Verification items for the finished model (mm, model axes). A direction names the side the tool comes from. Coordinates: 2 decimals unless noted, no trailing zeros. Write each loop counter-clockwise with the first axis right and the second up, starting at its lowest first coordinate (ties: lowest second). Pieces come first, ordered by that corner, then holes. Notation, with made-up numbers: (-20.75, 55) -> (33.25, 55) arc R14 cw to (33.25, 59) -> close; hole circle Ø11 at (78.5, 77). An arc over 180 degrees is marked (long way). Answer in a Markdown table with one row per item.
```python
from build123d import *

# Parameters (mm, degrees)
SKETCH_1_R      = 13.5
EXTRUDE_1_DEPTH = 2.5


with BuildPart() as part:
    # 草图1 → 凸台-拉伸1 (new body)
    with BuildSketch(Plane(origin=(0, 0, 0), x_dir=(1, 0, 0), z_dir=(0, 1, 0))):
        with Locations(Location((0, 0, 0), (0, 0, 90))):
            Circle(SKETCH_1_R)
        Polygon((0, -6.119912853), (5.3, -3.059956427), (5.3, 3.059956427), (0, 6.119912853), (-5.3, 3.059956427), (-5.3, -3.059956427), align=None, mode=Mode.SUBTRACT)
    extrude(amount=EXTRUDE_1_DEPTH)


solid = part.part
```
1. Sectioned sample at A-A, the plane z = 0. Record the cut outline in (x, y).
Findings below:
| item | result |
|---|---|
| outline | (-13.5, 0) -> (-5.3, 0) -> (-5.3, 2.5) -> (-13.5, 2.5) -> close; (5.3, 0) -> (13.5, 0) -> (13.5, 2.5) -> (5.3, 2.5) -> close |
2. Sectioned sample at C-C, the plane x = -1.5. Record the cut outline in (y, z).
Findings below:
| item | result |
|---|---|
| outline | (0, -13.42) -> (2.5, -13.42) -> (2.5, -5.25) -> (0, -5.25) -> close; (0, 5.25) -> (2.5, 5.25) -> (2.5, 13.42) -> (0, 13.42) -> close |
3. Release check for a two-part mould opening along Z. For faces 3 (the face through (-2.687, 1.232, 4.569)), 4 (the face through (6, 2.5, 0)), 5 (the face through (13.18, 1.23, 2.93)), 6 (the face through (-5.3, 1, 0)) record: released by +Z, released by -Z, zero draft, split by the parting line, or undercut.
Findings below:
| item | result |
|---|---|
| face 3 | undercut |
| face 4 | zero draft |
| face 5 | split by the parting line |
| face 6 | undercut |
4. Sectioned sample at B-B, the plane y = 1.05. Record the cut outline in (x, z).
Findings below:
| item | result |
|---|---|
| outline | circle Ø27 at (0, 0); hole (-5.3, -3.06) -> (0, -6.12) -> (5.3, -3.06) -> (5.3, 3.06) -> (0, 6.12) -> (-5.3, 3.06) -> close |
5. Sectioned sample at D-D, the plane x = 7.5. Record the cut outline in (y, z).
Findings below:
| item | result |
|---|---|
| outline | (0, -11.22) -> (2.5, -11.22) -> (2.5, 11.22) -> (0, 11.22) -> close |
6. Go/stop test with flat-tipped pins: pin 1 (0.8 mm diameter, centred on y = 0.5, z = 1, fed in from -X); pin 2 (0.8 mm diameter, centred on y = 1, z = 1.5, fed in from +X). Record where each tip stops, or that it passes through.
Findings below:
| item | result |
|---|---|
| pin 1 | stops at x = -13.49 |
| pin 2 | stops at x = 13.46 |
7. Material ranges on probe 1 along X at (y, z) = (1, 0.25); probe 2 along X at (y, z) = (2.05, -3.5); probe 3 along Z at (x, y) = (-1.5, 0.9), recorded low to high. Write a range as from..to.
Findings below:
| item | result |
|---|---|
| probe 1 | x = -13.5..-5.3, 5.3..13.5 |
| probe 2 | x = -13.04..-4.54, 4.54..13.04 |
| probe 3 | z = -13.42..-5.25, 5.25..13.42 |
8. Access from +Z, -Z, +X, -X, +Y, -Y to the whole of each face (thin tool, end or side, straight path). Record for faces 1 (the face through (-2.613, 1.232, -4.611)), 2 (the face through (6, 0, 0)).
Findings below:
| item | result |
|---|---|
| face 1 | +Y, -Y |
| face 2 | +Z, -Z, +X, -X, -Y |
